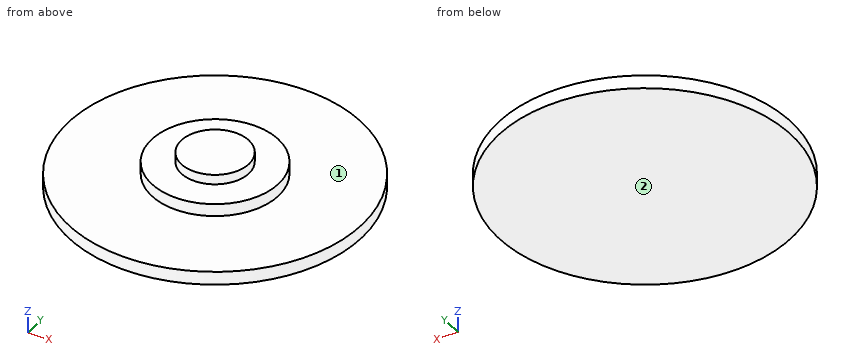
from build123d import *

# Parameters (mm, degrees)
F0_R     = 4.7625
F0_R_2   = 2.613606
F1_DEPTH = 1.9304
F0_R_3   = 11
F2_DEPTH = 1
F3_R     = 2.54
F4_DEPTH = 0.7366


with BuildPart() as f1:
    # F0 (on Top) → F1 (new body)
    with BuildSketch(Plane.XY):
        Circle(F0_R)
        Circle(F0_R_2, mode=Mode.SUBTRACT)
        Circle(F0_R_2)
    extrude(amount=F1_DEPTH)

    # F0 (on Top) → F2 (join)
    with BuildSketch(Plane.XY):
        Circle(F0_R_3)
        Circle(F0_R, mode=Mode.SUBTRACT)
    extrude(amount=F2_DEPTH)

    # F3 (on face) → F4 (join)
    with BuildSketch(Plane.XY.offset(1.9304)):
        Circle(F3_R)
    extrude(amount=F4_DEPTH)


solid = f1.part
For this review, take the finished solid that the model builds, in its own axes (mm). Face numbers are marked on the shaded views. A direction names the side the tool comes from. Round coordinates to 2 decimals unless told otherwise and drop trailing zeros. Write each loop counter-clockwise with the first axis right and the second up, starting at its lowest first coordinate (ties: lowest second). Pieces come first, ordered by that corner, then holes. Notation, with made-up numbers: M 37,-32.75 L 70,-32.75 A29 cw 70,-7.75 Z; hole C -32,-32.5 d7. An arc over 180 degrees is marked long. Write item = value, one per line. Start each with the question number.
(1) For line 1 along Z through (x, y) = (-4, -3.75); line 2 along X through (y, z) = (-4, 1.5); line 3 along Y through (x, z) = (-4.75, 0.85), list the stretches that pass through material, from the lowest coordinate up.
(2) We need section D-D (y = 3). Give the boundary of the cut face in (x, z), then the cut area to 3 significant figures.
(3) Clearance check with a flat-ended pin moving along its axis: pin 1 Ø1.5 at (x, y) = (6.5, -0.5) entering from +Z. State where the tip first meets the part, or that it passes through.
(4) For the marked faces 1 and 2, list the 3-axis set-ups (+Z, -Z, +X, -X, +Y, -Y) from which the entire face can be reached by the end or side of a thin tool; tool diameter is ignored.
(5) We need section A-A (y = 0). Give the boundary of the cut face in (x, z), then the cut area to 3 significant figures.
(6) We need section C-C (z = 0.6). Give the boundary of the cut face in (x, y).
Results found:
q1.line_1 = 0 to 1
q1.line_2 = -2.58 to 2.58
q1.line_3 = -9.92 to 9.92
q2.outline = M -10.58,0 L 10.58,0 L 10.58,1 L 3.7,1 L 3.7,1.93 L -3.7,1.93 L -3.7,1 L -10.58,1 Z
q2.area = 28.0 mm²
q3.pin_1 = 1
q4.face_1 = +Z
q4.face_2 = -Z, +X, -X, +Y, -Y
q5.outline = M -11,0 L 11,0 L 11,1 L 4.76,1 L 4.76,1.93 L 2.54,1.93 L 2.54,2.67 L -2.54,2.67 L -2.54,1.93 L -4.76,1.93 L -4.76,1 L -11,1 Z
q5.area = 34.6 mm²
q6.outline = C 0,0 d22
